from build123d import *

# Parameters (mm, degrees)
CROQUIS1_W              = 40
CROQUIS1_H              = 20
SALIENTE_EXTRUIR1_DEPTH = 12
REDONDEO1_R             = 4
CROQUIS2_R              = 2.5
CORTAR_EXTRUIR1_DEPTH   = 8
CROQUIS3_R              = 3.5
CORTAR_EXTRUIR2_DEPTH   = 10
CROQUIS4_R              = 2
CORTAR_EXTRUIR3_DEPTH   = 2


with BuildPart() as part:
    # Croquis1 → Saliente-Extruir1 (new body)
    with BuildSketch(Plane.XY):
        Rectangle(CROQUIS1_W, CROQUIS1_H)
    extrude(amount=SALIENTE_EXTRUIR1_DEPTH)

    # Redondeo1
    redondeo1_edges = [part.edges().sort_by_distance(p)[0] for p in [
        (20, -10, 6),
        (-20, -10, 6),
        (-20, 10, 6),
        (20, 10, 6),
    ]]
    fillet(redondeo1_edges, radius=REDONDEO1_R)

    # Croquis2 → Cortar-Extruir1 (cut)
    with BuildSketch(Plane(origin=(0, 0, 0), x_dir=(-1, 0, 0), z_dir=(0, 0, -1))):
        Circle(CROQUIS2_R)
    extrude(amount=-CORTAR_EXTRUIR1_DEPTH, mode=Mode.SUBTRACT)

    # Croquis3 → Cortar-Extruir2 (cut)
    with BuildSketch(Plane.XY.offset(12)):
        with Locations((-9.41266553, 0)):
            Circle(CROQUIS3_R)
        with Locations((9.41266553, 0)):
            Circle(CROQUIS3_R)
    extrude(amount=-CORTAR_EXTRUIR2_DEPTH, mode=Mode.SUBTRACT)

    # Croquis4 → Cortar-Extruir3 (cut)
    with BuildSketch(Plane.XY.offset(2)):
        with Locations((-9.41266553, 0)):
            Circle(CROQUIS4_R)
        with Locations((9.41266553, 0)):
            Circle(CROQUIS4_R)
    extrude(amount=-CORTAR_EXTRUIR3_DEPTH, mode=Mode.SUBTRACT)


solid = part.part
Here's how the part is built. I have some questions about the finished solid (model axes, mm). A direction names the side the tool comes from. Round coordinates to 2 decimals unless told otherwise and drop trailing zeros. Write each loop counter-clockwise with the first axis right and the second up, starting at its lowest first coordinate (ties: lowest second). Pieces come first, ordered by that corner, then holes.
1. I need wall thicknesses on L1, parallel to Y at x = 0, z = 2; L2, parallel to X at y = 1.75, z = 1.75; L3, parallel to X at y = 1, z = 0.5. Which ranges of each line are inside material? Lowest first, please.
2. Suppose I cut it at D-D (z = 11). List the corners of the cut face in (x, y) for me.
3. For faces 5 (the cylindrical face through (-7.565, -0.766, 1.014)), 6 (the flat face through (0, 0, 8)), 7 (the flat face through (11, -2, 2)), which set-ups out of +Z, -Z, +X, -X, +Y, -Y let a thin tool reach every point of the face, with its end or its side?
4. Will these pins go through, and if not, where does the flat tip stop? pin 1 Ø3 at (x, y) = (9.41, 0) entering from -Z; pin 2 Ø7.5 at (x, y) = (11, 1.5) entering from +Z; pin 3 Ø4.5 at (x, y) = (-9.41, 0) entering from +Z.
5. If we mould it in two halves opening along Y, with no side actions, what happens to faces 1 (the cylindrical face through (18.797, -8.859, 6.084)), 2 (the cylindrical face through (0.54, -2.44, 3.94)), 3 (the flat face through (0, 10, 6)), 4 (the flat face through (-20, 0, 6))? For each: released by +Y, released by -Y, zero draft, split by the parting line, or undercut.
6. Suppose I cut it at B-B (z = 7). List the corners of the cut face in (x, y) for me.
7. Suppose I cut it at A-A (y = 0). List the corners of the cut face in (x, z) for me.
8. Suppose I cut it at C-C (x = 9). List the corners of the cut face in (y, z) for me, and give its area (3 significant figures).
Answer sheet:
1. L1: y = -10 to -2.5, 2.5 to 10
1. L2: x = -20 to -10.38, -8.44 to -1.79, 1.79 to 8.44, 10.38 to 20
1. L3: x = -20 to -11.14, -7.68 to -2.29, 2.29 to 7.68, 11.14 to 20
2. outline: (-20, -6) arc R4 ccw to (-16, -10) - (16, -10) arc R4 ccw to (20, -6) - (20, 6) arc R4 ccw to (16, 10) - (-16, 10) arc R4 ccw to (-20, 6) - close; hole circle Ø7 at (-9.41, 0); hole circle Ø7 at (9.41, 0)
3. face 5: +Z, -Z
3. face 6: -Z
3. face 7: +Z
4. pin 1: passes through
4. pin 2: stops at z = 12
4. pin 3: stops at z = 2
5. face 1: released by -Y
5. face 2: undercut
5. face 3: released by +Y
5. face 4: zero draft
6. outline: (-20, -6) arc R4 ccw to (-16, -10) - (16, -10) arc R4 ccw to (20, -6) - (20, 6) arc R4 ccw to (16, 10) - (-16, 10) arc R4 ccw to (-20, 6) - close; hole circle Ø7 at (-9.41, 0); hole circle Ø5 at (0, 0); hole circle Ø7 at (9.41, 0)
7. outline: (-20, 0) - (-11.41, 0) - (-11.41, 2) - (-12.91, 2) - (-12.91, 12) - (-20, 12) - close; (-7.41, 0) - (-2.5, 0) - (-2.5, 8) - (2.5, 8) - (2.5, 0) - (7.41, 0) - (7.41, 2) - (5.91, 2) - (5.91, 12) - (-5.91, 12) - (-5.91, 2) - (-7.41, 2) - close; (11.41, 0) - (20, 0) - (20, 12) - (12.91, 12) - (12.91, 2) - (11.41, 2) - close
8. outline: (-10, 0) - (-1.96, 0) - (-1.96, 2) - (-3.48, 2) - (-3.48, 12) - (-10, 12) - close; (1.96, 0) - (10, 0) - (10, 12) - (3.48, 12) - (3.48, 2) - (1.96, 2) - close
8. area: 163 mm2
